For this review, use the dimensioned drawing (mm, ordinates from the lowest corner) and the shaded views. A direction names the side the tool comes from. Coordinates: 2 decimals unless noted, no trailing zeros. Order: outer loops, then holes, each group sorted by start corner. A loop starts at its lowest first (then second) coordinate and runs counter-clockwise, first axis right, second up. Notation, with made-up numbers: M -29.75,38.25 L -20.75,38.25 A6 cw -20.75,48.25 Z; hole C -8.5,1 d7. An arc over 180 degrees is marked long. Write each question's results on one line, items separated by ' | '.
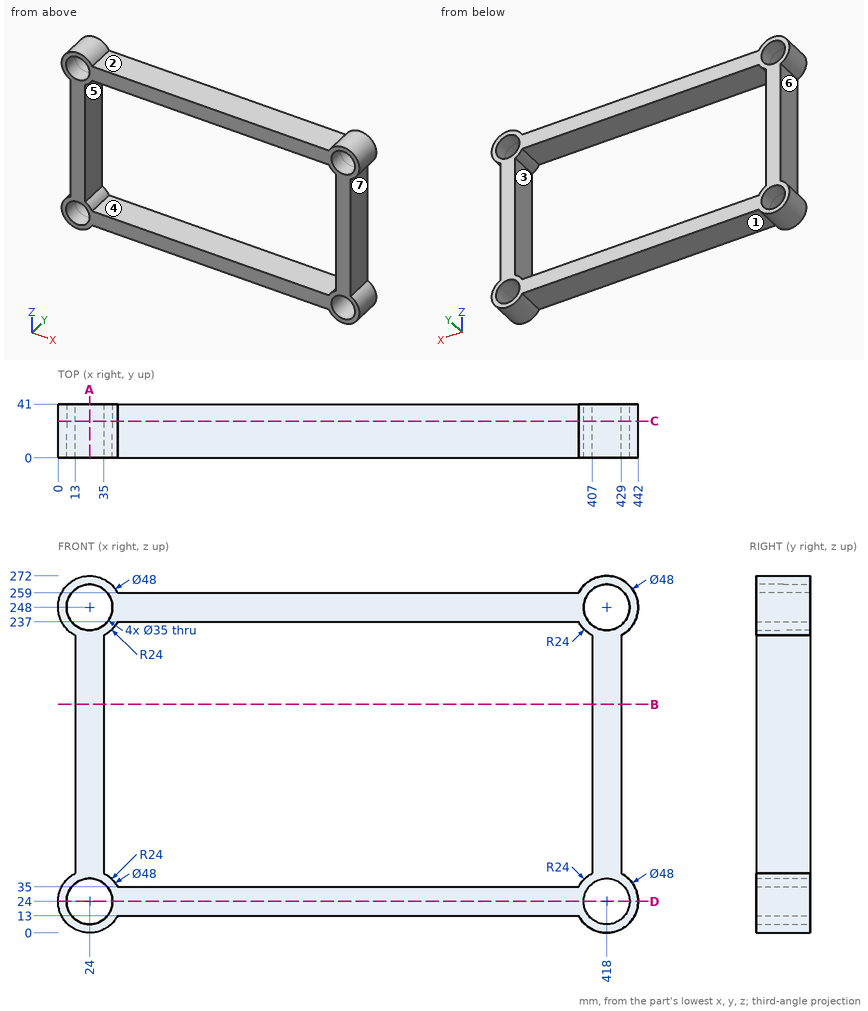
1) For the marked faces 5, 6 and 7, list the 3-axis set-ups (+Z, -Z, +X, -X, +Y, -Y) from which the entire face can be reached by the end or side of a thin tool; tool diameter is ignored.
Solutions:
face 5: +Y, -Y | face 6: -X, +Y, -Y | face 7: +X, +Y, -Y
2) Take a section at B-B on z = 174. State the section outline as (x, y) points, plus the area to 3 significant figures.
Solutions:
outline: M 13,0 L 35,0 L 35,41 L 13,41 Z; M 407,0 L 429,0 L 429,41 L 407,41 Z | area: 1,800 mm2
3) Take a section at A-A on x = 24. State the section outline as (y, z) points, plus the area to 3 significant figures.
Solutions:
outline: M 0,0 L 41,0 L 41,6.5 L 0,6.5 Z; M 0,41.5 L 41,41.5 L 41,230.5 L 0,230.5 Z; M 0,265.5 L 41,265.5 L 41,272 L 0,272 Z | area: 8,280 mm2
4) The part is to be moulded in two halves that separate along Z. For the marked faces 1, 2, 3 and 4, say which applies: pulls with the +Z half, pulls with the -Z half, needs draft (parallel to the pull), parting line crosses it, or undercut.
Solutions:
face 1: pulls with the -Z half | face 2: pulls with the +Z half | face 3: undercut | face 4: undercut
5) For pin 1 (1.5 mm diameter, centred on x = 167, y = 8, fed in from -Z); pin 2 (4 mm diameter, centred on x = 250, y = 15, fed in from +Z); pin 3 (12.5 mm diameter, centred on y = 22, z = 107.5, fed in from +X), all flat-tipped, find the tip position at first contact; note any pin that passes through.
Solutions:
pin 1: z = 13 | pin 2: z = 259 | pin 3: x = 429
6) To check wall thickness, follow line 1 along Z through (x, y) = (24, 33.5); line 2 along X through (y, z) = (15, 24); line 3 along X through (y, z) = (4, 177). State the ranges of each line that lie inside material, in increasing order.
Solutions:
line 1: 0 to 6.5, 41.5 to 230.5, 265.5 to 272 | line 2: 0 to 6.5, 41.5 to 400.5, 435.5 to 442 | line 3: 13 to 35, 407 to 429
7) Take a section at D-D on z = 24. State the section outline as (x, y) points.
Solutions:
outline: M 0,0 L 6.5,0 L 6.5,41 L 0,41 Z; M 41.5,0 L 400.5,0 L 400.5,41 L 41.5,41 Z; M 435.5,0 L 442,0 L 442,41 L 435.5,41 Z
8) Take a section at C-C on y = 28. State the section outline as (x, z) points.
Solutions:
outline: M 13,45.33 A24 ccw long 45.33,13 L 396.67,13 A24 ccw long 429,45.33 L 429,226.67 A24 ccw long 396.67,259 L 45.33,259 A24 ccw long 13,226.67 Z; hole C 24,24 d35; hole C 24,248 d35; hole M 35,45.33 A24 cw 45.33,35 L 396.67,35 A24 cw 407,45.33 L 407,226.67 A24 cw 396.67,237 L 45.33,237 A24 cw 35,226.67 Z; hole C 418,24 d35; hole C 418,248 d35
